Build history of the part. All positions in model axes, mm. A direction names the side the tool comes from. Give positions to 0.01 mm unless a question says otherwise; leave off trailing zeros. Loops run counter-clockwise (first coordinate to the right, second up) from the corner with the lowest first, then second, coordinate; pieces in that order, holes last. Notation, with made-up numbers: (-37, -14) -> (-2, -14) arc R22 cw to (-2, 18) -> close; hole circle Ø8 at (-23, -33.5). An arc over 180 degrees is marked (long way). Answer as a JSON object with one key per item and string values. Group by question number.
Q1. Wall check: probe 1 along X at (y, z) = (14.5, 23.5); probe 2 along Y at (x, z) = (-28.5, 77.5); probe 3 along Z at (x, y) = (77, 7). Give the ranges that are in metal, low to high. Write a range as from..to.
Q2. Band-saw the part on A-A, the plane z = 39. Write the cut outline in (x, y) (3 decimals), plus the area to 3 significant figures.
Q3. Drop flat-ended pins along their axis: pin 1 (12 mm diameter, centred on x = 37, z = 68, fed in from +Y); pin 2 (12.5 mm diameter, centred on x = 19.5, y = 19.5, fed in from -Z). Give the stop position or say it passes through.
Q4. Tool access for faces 1 (the flat face through (86.74, 15, 35)), 2 (the flat face through (-76, 27, -5.785)), 3 (the flat face through (89, 23, 24.24)): list every direction of +Z, -Z, +X, -X, +Y, -Y with a clear straight run to the whole face (end or side of a thin tool).
Q5. Band-saw the part on C-C, the plane z = 76. Write the cut outline in (x, y).
Q6. Band-saw the part on B-B, the plane x = -15.5. Write the cut outline in (y, z), plus the area to 3 significant figures.
Q7. Two-plate mould, pull along Y, no slides. Class faces 4 (the cylindrical face through (-8.48, 24.175, 84)), 5 (the flat face through (7, 17, -8.535)), 6 (the flat face through (5, 0, 36)): pulls with the +Y half, pulls with the -Y half, needs draft (parallel to the pull), parting line crosses it, or undercut.
from build123d import *

# Parameters (mm, degrees)
SKETCH3_W           = 170.58
SKETCH3_H           = 100
BOSS_EXTRUDE1_DEPTH = 5
SKETCH4_W           = 5
SKETCH4_H           = 100
BOSS_EXTRUDE2_DEPTH = 24.94
SKETCH6_W           = 160.58
SKETCH6_H           = 5
BOSS_EXTRUDE3_DEPTH = 24.94
BOSS_EXTRUDE4_DEPTH = 24.94
SKETCH8_R           = 1.75
CUT_EXTRUDE1_DEPTH  = 8
SKETCH9_W           = 7.75
SKETCH9_H           = 6.74
CUT_EXTRUDE2_DEPTH  = 10
SKETCH12_W          = 40.2
SKETCH12_H          = 14.565
CUT_EXTRUDE4_DEPTH  = 200
SKETCH13_R          = 1.75
CUT_EXTRUDE5_DEPTH  = 200
SKETCH14_R          = 1.75
CUT_EXTRUDE6_DEPTH  = 10


with BuildPart() as part:
    # Sketch3 → Boss-Extrude1 (new body)
    with BuildSketch(Plane(origin=(0, 0, 0), x_dir=(1, 0, 0), z_dir=(0, 1, 0))):
        with Locations((6.45008576, -36.464595487)):
            Rectangle(SKETCH3_W, SKETCH3_H)
    extrude(amount=BOSS_EXTRUDE1_DEPTH)

    # Sketch4 → Boss-Extrude2 (add)
    with BuildSketch(Plane(origin=(0, 5, 0), x_dir=(1, 0, 0), z_dir=(0, 1, 0))):
        with Locations((89.24008576, -36.464595487)):
            Rectangle(SKETCH4_W, SKETCH4_H)
        with Locations((-76.33991424, -36.464595487)):
            Rectangle(SKETCH4_W, SKETCH4_H)
    extrude(amount=BOSS_EXTRUDE2_DEPTH)

    # Sketch6 → Boss-Extrude3 (add)
    with BuildSketch(Plane(origin=(0, 5, 0), x_dir=(1, 0, 0), z_dir=(0, 1, 0))):
        with Locations((6.45008576, -83.964595487)):
            Rectangle(SKETCH6_W, SKETCH6_H)
    extrude(amount=BOSS_EXTRUDE3_DEPTH)

    # Sketch7 → Boss-Extrude4 (add)
    with BuildSketch(Plane(origin=(0, 5, 0), x_dir=(1, 0, 0), z_dir=(0, 1, 0))):
        Polygon((6.45008576, 13.535404513), (2.715085759, 13.535404513), (2.715085759, 8.535404513), (10.715085759, 8.535404513), (10.715085759, 13.535404513), align=None)
    extrude(amount=BOSS_EXTRUDE4_DEPTH)

    # Sketch8 → Cut-Extrude1 (cut)
    with BuildSketch(Plane.XY.offset(-8.535404513)):
        with Locations((6.715085759, 11.235)):
            Circle(SKETCH8_R)
        with Locations((6.715085759, 23.705)):
            Circle(SKETCH8_R)
    extrude(amount=-CUT_EXTRUDE1_DEPTH, mode=Mode.SUBTRACT)

    # Sketch9 → Cut-Extrude2 (cut)
    with BuildSketch(Plane.ZY.offset(78.83991424)):
        with Locations((-9.660404513, 26.57)):
            Rectangle(SKETCH9_W, SKETCH9_H)
    extrude(amount=-CUT_EXTRUDE2_DEPTH, mode=Mode.SUBTRACT)

    # Sketch12 → Cut-Extrude4 (cut)
    with BuildSketch(Plane.ZY.offset(78.83991424)):
        with Locations((44.339595487, 22.6575)):
            Rectangle(SKETCH12_W, SKETCH12_H)
    extrude(amount=-CUT_EXTRUDE4_DEPTH, mode=Mode.SUBTRACT)

    # Sketch13 → Cut-Extrude5 (cut)
    with BuildSketch(Plane.ZY.offset(78.83991424)):
        with Locations((69.23959554, 24.75)):
            Circle(SKETCH13_R)
        with Locations((19.43959554, 24.75)):
            Circle(SKETCH13_R)
    extrude(amount=-CUT_EXTRUDE5_DEPTH, mode=Mode.SUBTRACT)

    # Sketch14 → Cut-Extrude6 (cut)
    with BuildSketch(Plane.XY.offset(86.464595487)):
        with Locations((21.687920531, 22.44)):
            Circle(SKETCH14_R)
        with Locations((-8.252079469, 22.44)):
            Circle(SKETCH14_R)
        with Locations((77.74008576, 9)):
            Circle(SKETCH14_R)
    extrude(amount=-CUT_EXTRUDE6_DEPTH, mode=Mode.SUBTRACT)


solid = part.part
Worked answers:
{
 "1": {"probe 1": "-78.84..-73.84, 86.74..91.74", "probe 2": "0..5", "probe 3": "81.46..86.46"},
 "2": {"outline": "(-78.84, 0) -> (91.74, 0) -> (91.74, 15.375) -> (86.74, 15.375) -> (86.74, 5) -> (-73.84, 5) -> (-73.84, 15.375) -> (-78.84, 15.375) -> close", "area": "957 mm2"},
 "3": {"pin 1": "y = 5", "pin 2": "z = 81.46"},
 "4": {"face 1": "-Z, +Y", "face 2": "-Z, -X, +Y", "face 3": "+X, -X, +Y"},
 "5": {"outline": "(-78.84, 0) -> (91.74, 0) -> (91.74, 29.94) -> (86.74, 29.94) -> (86.74, 5) -> (-73.84, 5) -> (-73.84, 29.94) -> (-78.84, 29.94) -> close"},
 "6": {"outline": "(0, -13.54) -> (5, -13.54) -> (5, 81.46) -> (29.94, 81.46) -> (29.94, 86.46) -> (0, 86.46) -> close", "area": "625 mm2"},
 "7": {"face 4": "undercut", "face 5": "needs draft", "face 6": "pulls with the -Y half"}
}
